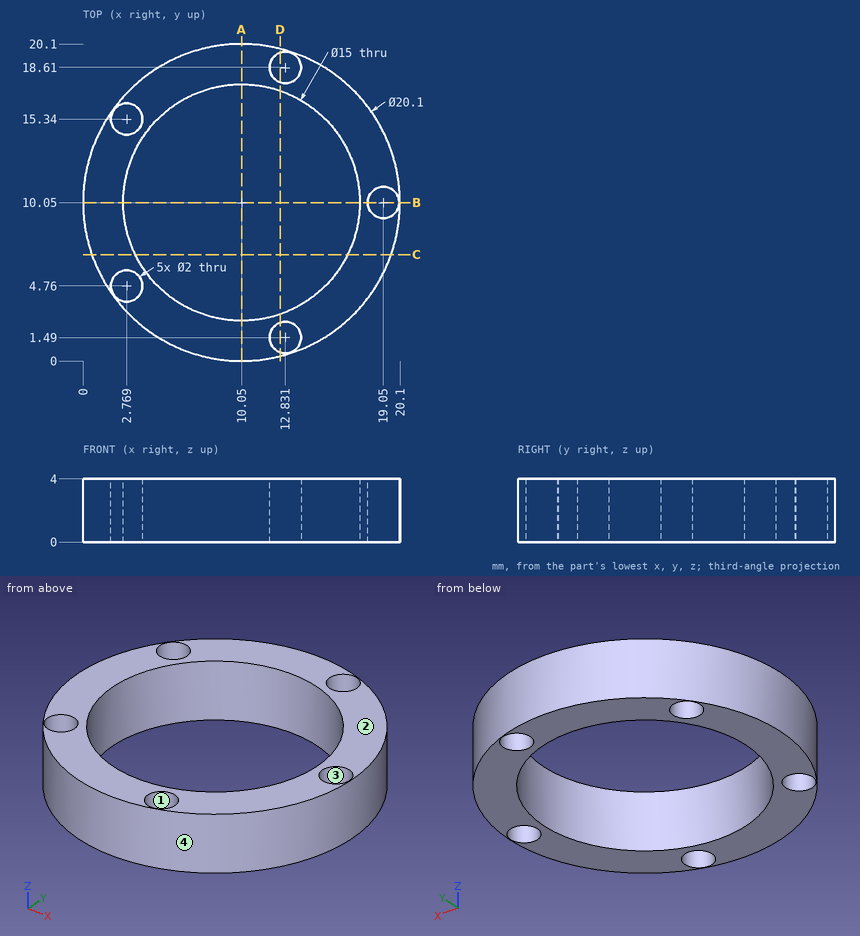
The drawing under review shows one solid part. Ordinate dimensions are in mm from its lowest x, y, z. Coordinates: 2 decimals unless noted, no trailing zeros. Loops run counter-clockwise (first coordinate to the right, second up) from the corner with the lowest first, then second, coordinate; pieces in that order, holes last. Notation, with made-up numbers: (-10.5, 6) - (-4.5, 6) arc R30 ccw to (-4.5, 44) - close; hole circle Ø4 at (-12.75, 52.5). An arc over 180 degrees is marked (long way). Return JSON: item names as keys, results as strings.
Item 1: Take a section at B-B (y = 10.05). Give the boundary of the cut face in (x, z), then the cut area to 3 significant figures.
Determined:
{"outline": "(0, 0) - (2.55, 0) - (2.55, 4) - (0, 4) - close; (17.55, 0) - (18.05, 0) - (18.05, 4) - (17.55, 4) - close; (20.05, 0) - (20.1, 0) - (20.1, 4) - (20.05, 4) - close", "area": "12.4 mm2"}
Item 2: Mouldability with a two-part tool opening along Y and no side actions: class the marked faces 1, 2, 3 and 4 as pulls with the +Y half, pulls with the -Y half, needs draft (parallel to the pull), parting line crosses it, or undercut.
Determined:
{"face 1": "undercut", "face 2": "needs draft", "face 3": "undercut", "face 4": "parting line crosses it"}
Item 3: Take a section at A-A (x = 10.05). Give the boundary of the cut face in (y, z), then the cut area to 3 significant figures.
Determined:
{"outline": "(0, 0) - (2.55, 0) - (2.55, 4) - (0, 4) - close; (17.55, 0) - (20.1, 0) - (20.1, 4) - (17.55, 4) - close", "area": "20.4 mm2"}
Item 4: Insertion check: pin 1 (12 mm diameter, centred on x = 10.5, y = 6.5, fed in from +Z); pin 2 (1 mm diameter, centred on x = 4.5, z = 2, fed in from +Y). Each pin has a flat end and moves straight along its axis. Give the tip position at first contact, or say it passes through.
Determined:
{"pin 1": "stops at z = 4", "pin 2": "stops at y = 18.74"}
Item 5: Take a section at D-D (x = 12.5). State how many separate pieces and enclosed holes the cut face has.
Determined:
{"separate pieces": "4", "enclosed holes": "0"}
Item 6: Take a section at C-C (y = 6.75). Give the boundary of the cut face in (x, z) (1 decimal).
Determined:
{"outline": "(0.6, 0) - (3.3, 0) - (3.3, 4) - (0.6, 4) - close; (16.8, 0) - (19.5, 0) - (19.5, 4) - (16.8, 4) - close"}
Item 7: For line 1 (Y direction, x = 10.25, z = 3.4); line 2 (Y direction, x = 3.5, z = 2.9) (1 decimal); line 3 (X direction, y = 6.5, z = 0.75) (1 decimal), list the stretches that pass through material, from the lowest coordinate up.
Determined:
{"line 1": "y = 0 to 2.55, 17.55 to 20.1", "line 2": "y = 2.4 to 4.1, 5.4 to 6.4, 13.7 to 14.7, 16 to 17.7", "line 3": "x = 0.6 to 3.4, 16.7 to 19.5"}
